Part model, mm, in its own coordinate system. A direction names the side the tool comes from. Coordinates: 2 decimals unless noted, no trailing zeros. Loops run counter-clockwise (first coordinate to the right, second up) from the corner with the lowest first, then second, coordinate; pieces in that order, holes last.
```python
from build123d import *

# Parameters (mm, degrees)
SKETCH_1_R            = 1.5
EXTRUDE_530_DEPTH     = 6
SKETCH_2_R            = 3
CUT_EXTRUDE_709_DEPTH = 3.3


with BuildPart() as part:
    # Эскиз1 → Extrude 530 (new body)
    with BuildSketch(Plane.XY):
        with BuildLine():
            Line((24, 3.3), (11.373653766, 3.3))
            ThreePointArc((11.373653766, 3.3), (7.909552151, 3.91916848), (4.874423043, 5.7))
            ThreePointArc((4.874423043, 5.7), (-7.5, 0), (4.874423043, -5.7))
            ThreePointArc((4.874423043, -5.7), (7.909552151, -3.91916848), (11.373653766, -3.3))
            Line((11.373653766, -3.3), (24, -3.3))
            ThreePointArc((24, -3.3), (27.3, 0), (24, 3.3))
        make_face()
        with Locations((24, 0)):
            Circle(SKETCH_1_R, mode=Mode.SUBTRACT)
        with Locations((20, 0)):
            Circle(SKETCH_1_R, mode=Mode.SUBTRACT)
        Circle(SKETCH_1_R, mode=Mode.SUBTRACT)
    extrude(amount=EXTRUDE_530_DEPTH)

    # Эскиз2 → Cut-Extrude 709 (cut)
    with BuildSketch(Plane.XY.offset(6)):
        Circle(SKETCH_2_R)
    extrude(amount=-CUT_EXTRUDE_709_DEPTH, mode=Mode.SUBTRACT)


solid = part.part
```
Q1. Drop flat-ended pins along their axis: P1, Ø1.5, axis at y = 2.5, z = 1.5, coming from the -X side; P2, Ø1.5, axis at y = 2.5, z = 4.5, coming from the +X side; P3, Ø1, axis at x = 17, z = 3.5, coming from the +Y side. Give the stop position or say it passes through.
Q2. Tool access for faces 4 (the flat face through (6, 0, 6)), 5 (the flat face through (1.3, -1.3, 2.7)), 6 (the flat face through (18, 3.3, 3)): list every direction of +Z, -Z, +X, -X, +Y, -Y with a clear straight run to the whole face (end or side of a thin tool).
Q3. Saw through at D-D (x = 0). List the corners of the cut face in (y, z).
Q4. Mould opens along X. For faces 1 (the flat face through (18, -3.3, 3)), 2 (the cylindrical face through (7.96, 3.9, 2.96)), 3 (the cylindrical face through (-3, 0, 4)) say: released by +X, released by -X, zero draft, split by the parting line, or undercut.
Q5. Probe line 1 (Y direction, x = 0, z = 3.75); line 2 (Y direction, x = 0, z = 1.4); line 3 (Y direction, x = 18, z = 0.45). List the from-to ranges inside material, lowest first.
Q6. Saw through at A-A (x = 20). List the corners of the cut face in (y, z).
Q7. Saw through at B-B (z = 3.3). List the corners of the cut face in (x, y), plus the area to 3 significant figures.
Q8. Saw through at C-C (y = 0). List the corners of the cut face in (x, z).
Checked values:
1. P1: stops at x = -7.29
1. P2: stops at x = 26.8
1. P3: stops at y = 3.3
2. face 4: +Z, +X, -X, +Y, -Y
2. face 5: +Z
2. face 6: +Z, -Z, +X, +Y
3. outline: (-7.5, 0) - (-1.5, 0) - (-1.5, 2.7) - (-3, 2.7) - (-3, 6) - (-7.5, 6) - close; (1.5, 0) - (7.5, 0) - (7.5, 6) - (3, 6) - (3, 2.7) - (1.5, 2.7) - close
4. face 1: zero draft
4. face 2: released by +X
4. face 3: undercut
5. line 1: y = -7.5 to -3, 3 to 7.5
5. line 2: y = -7.5 to -1.5, 1.5 to 7.5
5. line 3: y = -3.3 to 3.3
6. outline: (-3.3, 0) - (-1.5, 0) - (-1.5, 6) - (-3.3, 6) - close; (1.5, 0) - (3.3, 0) - (3.3, 6) - (1.5, 6) - close
7. outline: (4.87, -5.7) arc R10 cw to (11.37, -3.3) - (24, -3.3) arc R3.3 ccw to (24, 3.3) - (11.37, 3.3) arc R10 cw to (4.87, 5.7) arc R7.5 ccw (long way) to start; hole circle Ø6 at (0, 0); hole circle Ø3 at (20, 0); hole circle Ø3 at (24, 0)
7. area: 267 mm2
8. outline: (-7.5, 0) - (-1.5, 0) - (-1.5, 2.7) - (-3, 2.7) - (-3, 6) - (-7.5, 6) - close; (1.5, 0) - (18.5, 0) - (18.5, 6) - (3, 6) - (3, 2.7) - (1.5, 2.7) - close; (21.5, 0) - (22.5, 0) - (22.5, 6) - (21.5, 6) - close; (25.5, 0) - (27.3, 0) - (27.3, 6) - (25.5, 6) - close
